Verification items for the finished model (mm, model axes). A direction names the side the tool comes from. Coordinates: 2 decimals unless noted, no trailing zeros. Order: outer loops, then holes, each group sorted by start corner. A loop starts at its lowest first (then second) coordinate and runs counter-clockwise, first axis right, second up. Notation, with made-up numbers: (-28, 36.25) - (-22, 36.25) arc R15 ccw to (-22, 53.25) - close; hole circle Ø9 at (45, 54.5). An arc over 180 degrees is marked (long way). Answer as CSV lines item,"result". Start each with the question number.
1. Material ranges on L1, parallel to X at y = -0.75, z = -35; L2, parallel to Y at x = 31, z = -31.5; L3, parallel to Z at x = 63.5, y = -5.5, recorded low to high. Write a range as [from, to].
2. Section check C-C (z = -37). Record the cut outline in (x, y).
3. Mould release check, pull along X, two halves, no side actions. Record for faces 1 (the flat face through (46.86, 0.79, 1.01)), 2 (the flat face through (12.992, -4, -28)), 3 (the flat face through (3.812, -4, -28)), 4 (the flat face through (8, 6, -5.031)): pulls with the +X half, pulls with the -X half, needs draft (parallel to the pull), parting line crosses it, or undercut.
4. Set-up check for faces 5 (the flat face through (60, 6, -5.031)), 6 (the flat face through (60, -4, -49.001)), 7 (the flat face through (60, -4, -5.031)), 8 (the flat face through (8, 6, -51.544)), 9 (the flat face through (65.608, 6, -27)): record each of +Z, -Z, +X, -X, +Y, -Y from which the full face is reachable in a straight line by a thin tool's end or side.
5. Section check A-A (x = 59.13). Record the cut outline in (y, z), and give its area (3 significant figures).
6. Go/stop test with flat-tipped pins: pin 1 (3 mm diameter, centred on x = 47, z = -52, fed in from +Y); pin 2 (4 mm diameter, centred on y = -2.5, z = -31, fed in from -X); pin 3 (4 mm diameter, centred on y = 7.5, z = -32, fed in from +X); pin 4 (8 mm diameter, centred on y = -5.5, z = -59.5, fed in from +X). Record where each tip stops, or that it passes through.
7. Section check B-B (y = -2). Record the cut outline in (x, z).
8. Section check D-D (x = 43.89). Record the cut outline in (y, z).
from build123d import *

# Parameters (mm, degrees)
SKETCH1_R                = 1.5
BOSS_EXTRUDE1_DEPTH      = 1.6
BOSS_EXTRUDE2_DEPTH      = 8
BOSS_EXTRUDE2_DEPTH_BACK = 9.6
SKETCH2_W                = 9.179453462
SKETCH2_H                = 46.512773029
SKETCH2_W_2              = 10.081020205
SKETCH2_H_2              = 43.969790628


with BuildPart() as part:
    # Sketch1 → Boss-Extrude1 (new body)
    with BuildSketch(Plane(origin=(0, 0, 0), x_dir=(1, 0, 0), z_dir=(0, 1, 0))):
        Polygon((0, 0), (10.87, 0), (12.87, -2), (45.87, -2), (47.87, 0), (70, 0), (70, 80.5), (0, 80.5), align=None)
        with Locations(Location((10.87, 55.61, 0), (0, 0, 270))):
            Circle(SKETCH1_R, mode=Mode.SUBTRACT)
        with Locations(Location((59.13, 53.84, 0), (0, 0, 270))):
            Circle(SKETCH1_R, mode=Mode.SUBTRACT)
        with Locations(Location((43.89, 0, 0), (0, 0, 270))):
            Circle(SKETCH1_R, mode=Mode.SUBTRACT)
    extrude(amount=BOSS_EXTRUDE1_DEPTH)

    # Sketch2 → Boss-Extrude2 (add, two sides: drawn at the far end of the back side and taken through both)
    with BuildSketch(Plane(origin=(0, 1.6, 0), x_dir=(1, 0, 0), z_dir=(0, 1, 0)).offset(-BOSS_EXTRUDE2_DEPTH_BACK)):
        with Locations((8.40218686, 28.287509228)):
            Rectangle(SKETCH2_W, SKETCH2_H)
        with Locations((60.567754225, 27.016018028)):
            Rectangle(SKETCH2_W_2, SKETCH2_H_2)
    extrude(amount=BOSS_EXTRUDE2_DEPTH + BOSS_EXTRUDE2_DEPTH_BACK)


solid = part.part
Evaluation:
1,L1,"x = [3.81, 12.99], [55.53, 65.61]"
1,L2,"y = [0, 1.6]"
1,L3,"z = [-49, -5.03]"
2,outline,"(0, 0) - (3.81, 0) - (3.81, -8) - (12.99, -8) - (12.99, 0) - (55.53, 0) - (55.53, -8) - (65.61, -8) - (65.61, 0) - (70, 0) - (70, 1.6) - (65.61, 1.6) - (65.61, 9.6) - (55.53, 9.6) - (55.53, 1.6) - (12.99, 1.6) - (12.99, 9.6) - (3.81, 9.6) - (3.81, 1.6) - (0, 1.6) - close"
3,face 1,"pulls with the +X half"
3,face 2,"undercut"
3,face 3,"pulls with the -X half"
3,face 4,"needs draft"
4,face 5,"+Z, +X, -X, +Y"
4,face 6,"-Z, +X, -Y"
4,face 7,"+Z, +X, -X, -Y"
4,face 8,"-Z, +X, -X, +Y"
4,face 9,"+Z, -Z, +X, +Y"
5,outline,"(-8, -49) - (0, -49) - (0, -52.34) - (1.6, -52.34) - (1.6, -49) - (9.6, -49) - (9.6, -5.03) - (1.6, -5.03) - (1.6, 0) - (0, 0) - (0, -5.03) - (-8, -5.03) - close; (0, -80.5) - (1.6, -80.5) - (1.6, -55.34) - (0, -55.34) - close"
5,area,"828 mm²"
6,pin 1,"stops at y = 1.6"
6,pin 2,"stops at x = 3.81"
6,pin 3,"stops at x = 65.61"
6,pin 4,"passes through"
7,outline,"(3.81, -51.54) - (12.99, -51.54) - (12.99, -5.03) - (3.81, -5.03) - close; (55.53, -49) - (65.61, -49) - (65.61, -5.03) - (55.53, -5.03) - close"
8,outline,"(0, -80.5) - (1.6, -80.5) - (1.6, -1.5) - (0, -1.5) - close; (0, 1.5) - (1.6, 1.5) - (1.6, 2) - (0, 2) - close"
